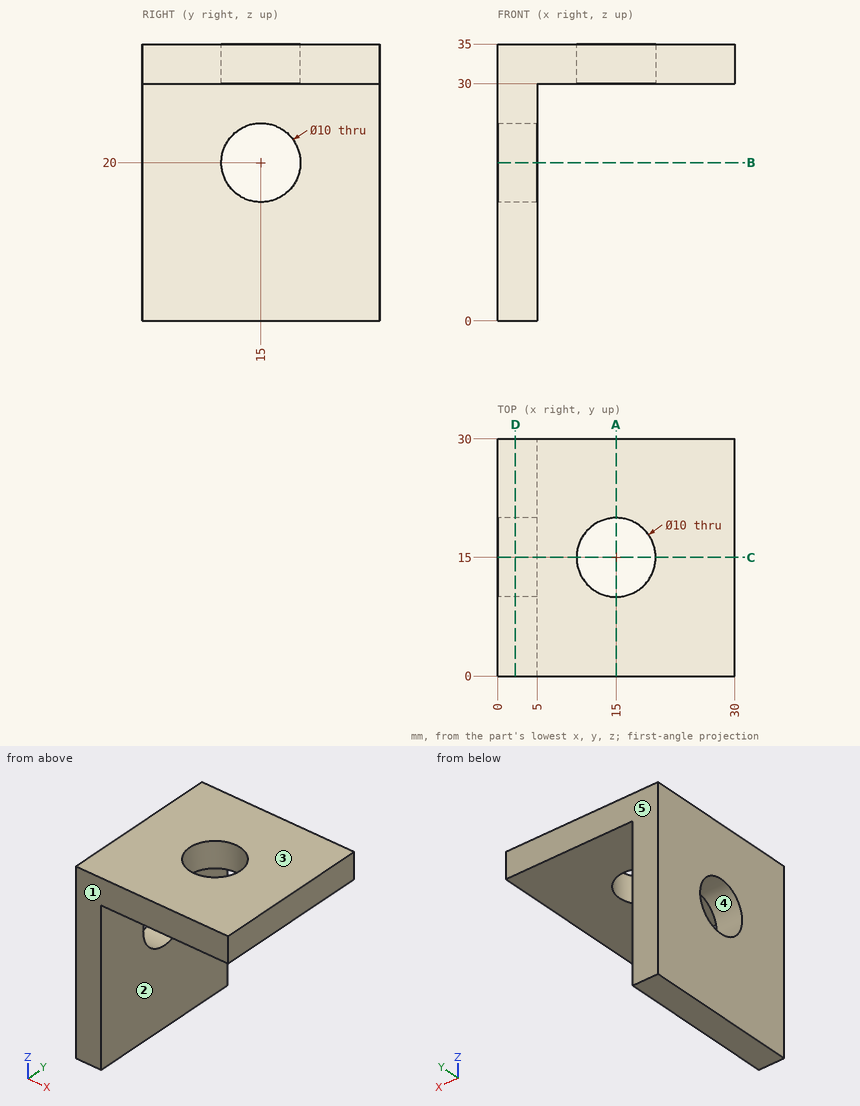
Part print with two shaded views. Sizes in mm from the minimum x, y, z corner. A direction names the side the tool comes from. Coordinates: 2 decimals unless noted, no trailing zeros. Write each loop counter-clockwise with the first axis right and the second up, starting at its lowest first coordinate (ties: lowest second). Pieces come first, ordered by that corner, then holes.
(1) Cut at B-B on z = 20. List the corners of the cut face in (x, y).
(2) Cut at A-A on x = 15. List the corners of the cut face in (y, z).
(3) 3-axis set-ups, long thin cutter, end or side, ignore diameter. For the marked faces 1 and 2: which of +Z, -Z, +X, -X, +Y, -Y reach the whole face in a straight line?
(4) Cut at C-C on y = 15. List the corners of the cut face in (x, z), and give its area (3 significant figures).
(5) Drill centre lines: line 1 (Y direction, x = 1.55, z = 20); line 2 (X direction, y = 10.5, z = 23.5); line 3 (Z direction, x = 16, y = 22.25). Where is each one in solid material? Low to high.
(6) Pin check, flat tips, straight feed: pin 1 Ø12 at (x, y) = (26, 9) entering from -Z; pin 2 Ø1.5 at (y, z) = (27, 18.5) entering from -X; pin 3 Ø15 at (y, z) = (11.5, 14) entering from +X. Stop position of each tip, or through.
(7) Mould opens along Z. For the marked faces 3, 4 and 5 say: pulls with the +Z half, pulls with the -Z half, needs draft (parallel to the pull), parting line crosses it, or undercut.
(8) Cut at D-D on x = 2.25. List the corners of the cut face in (y, z).
Working result:
1. outline: (0, 0) - (5, 0) - (5, 10) - (0, 10) - close; (0, 20) - (5, 20) - (5, 30) - (0, 30) - close
2. outline: (0, 30) - (10, 30) - (10, 35) - (0, 35) - close; (20, 30) - (30, 30) - (30, 35) - (20, 35) - close
3. face 1: +Z, -Z, +X, -X, -Y
3. face 2: -Z, +X, +Y, -Y
4. outline: (0, 0) - (5, 0) - (5, 15) - (0, 15) - close; (0, 25) - (5, 25) - (5, 30) - (10, 30) - (10, 35) - (0, 35) - close; (20, 30) - (30, 30) - (30, 35) - (20, 35) - close
4. area: 200 mm2
5. line 1: y = 0 to 10, 20 to 30
5. line 2: x = 0 to 5
5. line 3: z = 30 to 35
6. pin 1: stops at z = 30
6. pin 2: stops at x = 0
6. pin 3: stops at x = 5
7. face 3: pulls with the +Z half
7. face 4: undercut
7. face 5: needs draft
8. outline: (0, 0) - (30, 0) - (30, 35) - (0, 35) - close; hole circle Ø10 at (15, 20)
